Could you check a few things on this drawing? It's one solid part, dimensions in mm from its lowest x, y, z. A direction names the side the tool comes from. Round coordinates to 2 decimals unless told otherwise and drop trailing zeros. Loops run counter-clockwise (first coordinate to the right, second up) from the corner with the lowest first, then second, coordinate; pieces in that order, holes last. Notation, with made-up numbers: M 39.5,76 L 74.5,76 A5 ccw 74.5,85 Z; hole C 1,5 d4. An arc over 180 degrees is marked long. Write item = value, one per line. Start each with the question number.
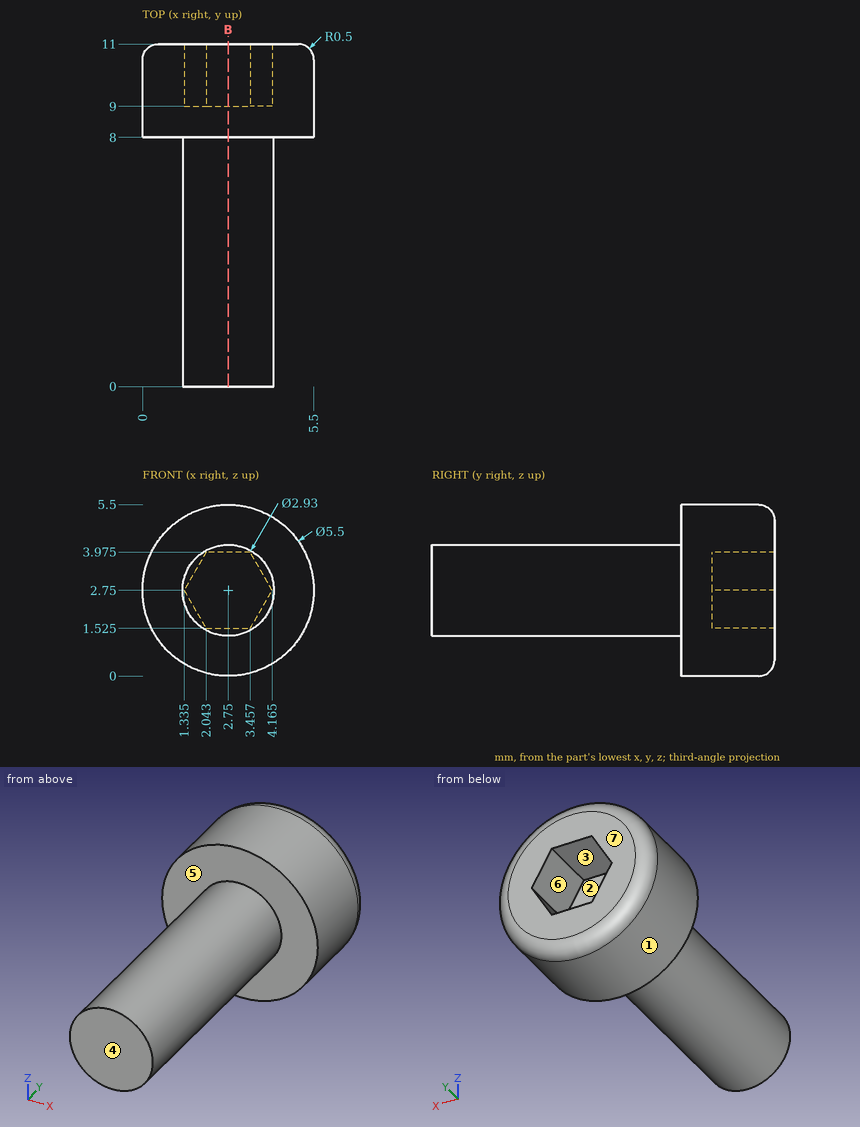
Item 1: I want a section at B-B, the plane x = 2.75. List the corners of the cut face in (y, z) for me (1 decimal).
Item 2: Will these pins go through, and if not, where does the flat tip stop? pin 1 Ø2 at (y, z) = (6.5, 4.5) entering from -X; pin 2 Ø1 at (y, z) = (5, 1) entering from -X (1 decimal); pin 3 Ø0.7 at (x, z) = (3, 3) entering from +Y.
Item 3: For the marked faces 5, 6 and 7, which set-ups out of +Z, -Z, +X, -X, +Y, -Y let a thin tool reach every point of the face, with its end or its side?
Item 4: We'd pull the mould along X, two halves only. Please class the marked faces 1, 2, 3 and 4: released by +X, released by -X, zero draft, split by the parting line, or undercut.
Item 5: Please list where these lines run through material, in increasing order: line 1 (Y direction, x = 3.2, z = 2.8); line 2 (Y direction, x = 5.05, z = 2.6); line 3 (X direction, y = 6.75, z = 2.7) (1 decimal). Write a range as [from, to].
Worked out:
q1.outline = M 0,1.3 L 8,1.3 L 8,0 L 10.5,0 A0.5 ccw 11,0.5 L 11,1.5 L 9,1.5 L 9,4 L 11,4 L 11,5 A0.5 ccw 10.5,5.5 L 8,5.5 L 8,4.2 L 0,4.2 Z
q2.pin_1 = 1.49
q2.pin_2 = 2
q2.pin_3 = 9
q3.face_5 = -Y
q3.face_6 = +Y
q3.face_7 = +Z, -Z, +X, -X, +Y
q4.face_1 = split by the parting line
q4.face_2 = undercut
q4.face_3 = undercut
q4.face_4 = zero draft
q5.line_1 = [0, 9]
q5.line_2 = [8, 11]
q5.line_3 = [1.3, 4.2]
